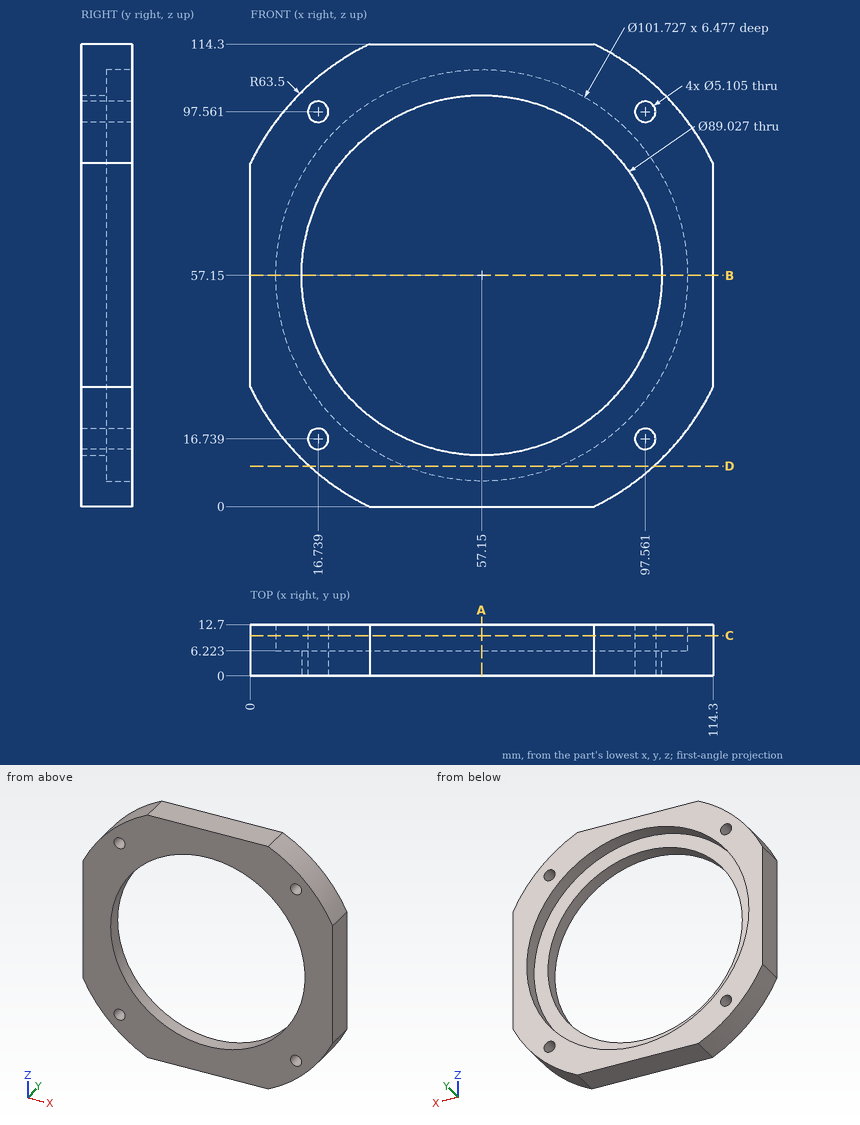
Design review of the part shown in the three views and the two pictorial views. Dimensions are in mm from the part's minimum x, y and z. Round coordinates to 2 decimals unless told otherwise and drop trailing zeros. Write each loop counter-clockwise with the first axis right and the second up, starting at its lowest first coordinate (ties: lowest second). Pieces come first, ordered by that corner, then holes. Notation, with made-up numbers: M 17,12.25 L 22,12.25 A18 ccw 22,34.25 Z; hole C 45.5,-11 d3. An arc over 180 degrees is marked long. One line per item, written item: value. Start each with the question number.
1. Take a section at C-C on y = 10. State how many separate pieces and enclosed holes the cut face has, then the cut area to 3 significant figures.
2. Clearance check with flat-ended pins moving along their axes: P1, Ø4, axis at x = 94, z = 101, coming from the -Y side; P2, Ø10, axis at x = 68.5, z = 18, coming from the +Y side; P3, Ø3, axis at x = 16.74, z = 97.56, coming from the +Y side. State where each tip first meets the part, or that it passes through.
3. To check wall thickness, follow probe 1 along Z at (x, y) = (57.15, 11.75); probe 2 along Z at (x, y) = (15, 11.5) (1 decimal); probe 3 along Y at (x, z) = (78, 12). State the ranges of each line that lie inside material, in increasing order. Write a range as from..to.
4. Take a section at D-D on z = 10. State the section outline as (x, y) points.
5. Take a section at B-B on z = 57.15. State the section outline as (x, y) points.
6. Take a section at A-A on x = 57.15. State the section outline as (y, z) points.
Computed:
1. separate pieces: 1
1. enclosed holes: 5
1. area: 3,510 mm²
2. P1: stops at y = 0
2. P2: stops at y = 6.22
2. P3: passes through
3. probe 1: z = 0..6.29, 108.01..114.3
3. probe 2: z = 9.7..14.9, 18.6..28.7, 85.6..95.7, 99.4..104.6
3. probe 3: y = 0..6.22
4. outline: M 14.62,0 L 99.68,0 L 99.68,12.7 L 76.23,12.7 L 76.23,6.22 L 38.07,6.22 L 38.07,12.7 L 14.62,12.7 Z
5. outline: M 0,0 L 12.64,0 L 12.64,6.22 L 6.29,6.22 L 6.29,12.7 L 0,12.7 Z; M 101.66,0 L 114.3,0 L 114.3,12.7 L 108.01,12.7 L 108.01,6.22 L 101.66,6.22 Z
6. outline: M 0,0 L 12.7,0 L 12.7,6.29 L 6.22,6.29 L 6.22,12.64 L 0,12.64 Z; M 0,101.66 L 6.22,101.66 L 6.22,108.01 L 12.7,108.01 L 12.7,114.3 L 0,114.3 Z
